Autodesk Inventor part; units mm, degrees
ref_plane "YZ Plane" through (0, 0, 0) normal (1, 0, 0) x (0, 1, 0)
ref_plane "XZ Plane" through (0, 0, 0) normal (0, 1, 0) x (-1, 0, 0)
ref_plane "XY Plane" through (0, 0, 0) normal (0, 0, 1) x (1, 0, 0)
sketch "Schizzo1" plane through (0, 0, 0) normal (0, 1, 0) x (-1, 0, 0)
  line L0 (-67.55, 63) -> (67.55, 63)
  line L1 (67.55, 63) -> (67.55, -63)
  line L2 (67.55, -63) -> (-67.55, -63)
  line L3 (-67.55, -63) -> (-67.55, 63)
  line L4 (-67.55, 63) -> (67.55, -63) construction
  line L5 (67.55, 63) -> (-67.55, -63) construction
  line L6 (67.55, -55.2) -> (43.733, -55.2) construction
  line L7 (43.733, -55.2) -> (-36.267, -55.2) construction
  line L8 (-36.267, -55.2) -> (-36.267, -42.3) construction
  line L9 (-36.267, -42.3) -> (43.733, -42.3) construction
  line L10 (43.733, -42.3) -> (43.733, -55.2) construction
  line L11 (-36.267, 63) -> (-36.267, 55.2) construction
  line L12 (-36.267, 55.2) -> (43.733, 55.2) construction
  line L13 (43.733, 55.2) -> (43.733, 42.3) construction
  line L14 (43.733, 42.3) -> (-36.267, 42.3) construction
  line L15 (-36.267, 42.3) -> (-36.267, 55.2) construction
  line L16 (-36.267, -48.75) -> (-31.267, -48.75) construction
  circle A0 centre (-31.267, -48.75) radius 2
  line L17 (-31.267, -48.75) -> (-16.267, -48.75) construction
  circle A1 centre (-16.267, -48.75) radius 2
  line L18 (43.733, 48.75) -> (38.733, 48.75) construction
  circle A2 centre (38.733, 48.75) radius 2
  line L19 (38.733, 48.75) -> (23.733, 48.75) construction
  circle A3 centre (23.733, 48.75) radius 2
  line L20 (-31.267, -63) -> (-31.267, -55.2) construction
  point P0 (0, 0)
  dimension "d0" = 135.1
  dimension "d1" = 126
  dimension "d18" = 23.817
  dimension "d19" = 80
  dimension "d20" = 12.9
  dimension "d21" = 7.8
  dimension "d22" = 12.9
  dimension "d23" = 5
  dimension "d24" = 31.283
  dimension "d26" = 4
  dimension "d27" = 15
  dimension "d28" = 4
  dimension "d37" = 5
  dimension "d38" = 4
  dimension "d39" = 15
  dimension "d40" = 4
  dimension "d55" = 7.8
extrude "Estrusione1" add sketch "Schizzo1" along normal blind 5 contours L0 L1 L2 L3 | A0 | A1 | A2 | A3
hole "Foro3" at (16.267, 0, -48.75) at (31.267, 0, -48.75) at (-23.733, 0, 48.75) at (-38.733, 0, 48.75) direction (0, 1, 0) diameter 4 depth 10 countersink diameter 6 countersink angle 90
properties part number "PiattoBilancia"
The model under review builds one solid part; all positions refer to its coordinate system, in mm. Round coordinates to 2 decimals unless told otherwise and drop trailing zeros. Loops run counter-clockwise (first coordinate to the right, second up) from the corner with the lowest first, then second, coordinate; pieces in that order, holes last. Notation, with made-up numbers: M 14,53.25 L 58,53.25 A26 cw 58,72.25 Z; hole C 21.5,79.5 d9. An arc over 180 degrees is marked long. Answer as a JSON object with one key per item and string values.
(1) To check wall thickness, follow line 1 along X through (y, z) = (2.65, -48.75); line 2 along Z through (x, y) = (32.5, 2.2); line 3 along Z through (x, y) = (33, 0.25). State the ranges of each line that lie inside material, in increasing order.
Resolved:
{"line 1": "-67.55 to 14.27, 18.27 to 29.27, 33.27 to 67.55", "line 2": "-63 to -50.32, -47.18 to 63", "line 3": "-63 to -50.89, -46.61 to 63"}
(2) Take a section at A-A on z = -48.75. Give the boundary of the cut face in (x, y).
Resolved:
{"outline": "M -67.55,0 L 13.27,0 L 14.27,1 L 14.27,5 L -67.55,5 Z; M 18.27,1 L 19.27,0 L 28.27,0 L 29.27,1 L 29.27,5 L 18.27,5 Z; M 33.27,1 L 34.27,0 L 67.55,0 L 67.55,5 L 33.27,5 Z"}
(3) Draft analysis for pull direction Z (two halves, no side actions). For faces 1 (the cylindrical face through (-25.716, 3.028, 49.01)), 2 (the cylindrical face through (-40.716, 3.028, 49.01)), 3 (the flat face through (1, 0, 1)), 4 (the flat face through (1, 2, 63)), state which applies: released by +Z, released by -Z, zero draft, split by the parting line, or undercut.
Resolved:
{"face 1": "undercut", "face 2": "undercut", "face 3": "zero draft", "face 4": "released by +Z"}
